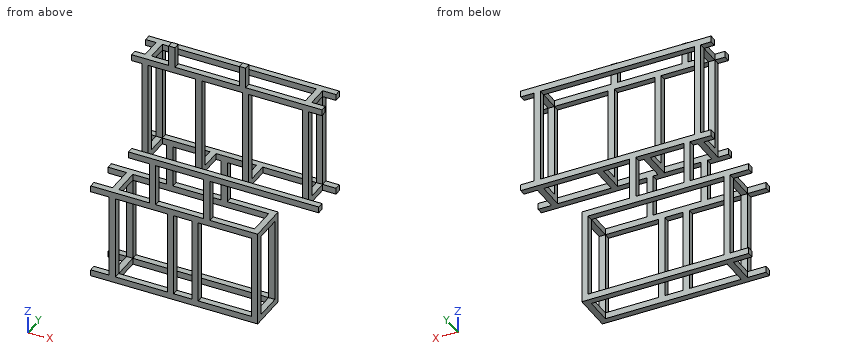
from build123d import *

# Parameters (mm, degrees)
SKETCH_1_W          = 30
SKETCH_1_H          = 450
SKETCH_1_W_2        = 910
SKETCH_1_H_2        = 30
EXTRUDE_1_DEPTH     = 30
SKETCH_2_W          = 30.109824799
SKETCH_2_H          = 30
SKETCH_2_W_2        = 30
EXTRUDE_2_DEPTH     = 100
SKETCH_3_W          = 49.418401049
SKETCH_3_H          = 30
SKETCH_3_W_2        = 30
SKETCH_3_W_3        = 910
SKETCH_3_H_2        = 450
EXTRUDE_3_DEPTH     = 30
SKETCH_4_W          = 850
SKETCH_4_H          = 30
SKETCH_4_W_2        = 30
SKETCH_4_H_2        = 400
EXTRUDE_4_DEPTH     = 30
SKETCH_5_W          = 30
SKETCH_5_H          = 30
EXTRUDE_5_DEPTH     = 130
SKETCH_6_W          = 88.479210194
SKETCH_6_H          = 30
SKETCH_6_W_2        = 30
SKETCH_6_H_2        = 400
SKETCH_6_W_3        = 850
EXTRUDE_6_DEPTH     = 30
SKETCH_8_W          = 736.515263892
SKETCH_8_H          = 30
SKETCH_8_W_2        = 64.066335059
SKETCH_8_W_3        = 49.418401049
CUT_EXTRUDE_2_DEPTH = 30
SKETCH_9_W          = 910
SKETCH_9_H          = 30
EXTRUDE_7_DEPTH     = 30
SKETCH_12_W         = 30
SKETCH_12_H         = 130
EXTRUDE_8_DEPTH     = 30
SKETCH_13_W         = 30
SKETCH_13_H         = 200
EXTRUDE_9_DEPTH     = 30
SKETCH_14_W         = 30
SKETCH_14_H         = 200
EXTRUDE_10_DEPTH    = 30
SKETCH_15_W         = 489.531957018
SKETCH_15_H         = 254.722560686
CUT_EXTRUDE_3_DEPTH = 51.972649134
SKETCH_16_W         = 30
SKETCH_16_H         = 30
EXTRUDE_11_DEPTH    = 100


with BuildPart() as part:
    # Sketch 1 → Extrude 1 (new body)
    with BuildSketch(Plane(origin=(0, 0, 0), x_dir=(1, 0, 0), z_dir=(0, 1, 0))):
        with Locations((64.418401049, 255)):
            Rectangle(SKETCH_1_W, SKETCH_1_H)
        with Locations((455, 15)):
            Rectangle(SKETCH_1_W_2, SKETCH_1_H_2)
        with Locations((321.408548695, 255)):
            Rectangle(SKETCH_1_W, SKETCH_1_H)
        with Locations((544.693031268, 255)):
            Rectangle(SKETCH_1_W, SKETCH_1_H)
        with Locations((830.933664941, 255)):
            Rectangle(SKETCH_1_W, SKETCH_1_H)
        Polygon((0, 480), (49.418401049, 480), (79.418401049, 480), (306.408548695, 480), (336.408548695, 480), (529.693031268, 480), (559.693031268, 480), (815.933664941, 480), (845.933664941, 480), (910, 480), (910, 510), (0, 510), align=None)
    extrude(amount=EXTRUDE_1_DEPTH)

    # Sketch 2 → Extrude 2 (add)
    with BuildSketch(Plane(origin=(0, 30, 0), x_dir=(1, 0, 0), z_dir=(0, 1, 0))):
        with Locations((64.473313449, 15)):
            Rectangle(SKETCH_2_W, SKETCH_2_H)
        with Locations((830.933664941, 15)):
            Rectangle(SKETCH_2_W_2, SKETCH_2_H)
        with Locations((64.418401049, 495)):
            Rectangle(SKETCH_2_W_2, SKETCH_2_H)
        with Locations((830.933664941, 495)):
            Rectangle(SKETCH_2_W_2, SKETCH_2_H)
    extrude(amount=EXTRUDE_2_DEPTH)

    # Sketch 3 → Extrude 3 (add)
    with BuildSketch(Plane(origin=(0, 130, 0), x_dir=(1, 0, 0), z_dir=(0, 1, 0))):
        Polygon((910, 510), (79.418401049, 510), (79.418401049, 480), (79.528225848, 480), (815.933664941, 480), (845.933664941, 480), (910, 480), align=None)
        with Locations((24.709200525, 495)):
            Rectangle(SKETCH_3_W, SKETCH_3_H)
        with Locations((64.418401049, 495)):
            Rectangle(SKETCH_3_W_2, SKETCH_3_H)
        with Locations((455, 15)):
            Rectangle(SKETCH_3_W_3, SKETCH_3_H)
        Polygon((79.418401049, 480), (49.418401049, 480), (49.418401049, 30), (79.528225848, 30), (79.528225848, 480), align=None)
        with Locations((830.933664941, 255)):
            Rectangle(SKETCH_3_W_2, SKETCH_3_H_2)
    extrude(amount=EXTRUDE_3_DEPTH)

    # Sketch 8 → Cut-Extrude 2 (cut)
    with BuildSketch(Plane(origin=(0, 0, -510), x_dir=(-1, 0, 0), z_dir=(0, 0, -1))):
        with Locations((-447.676032995, 15)):
            Rectangle(SKETCH_8_W, SKETCH_8_H)
        with Locations((-877.966832471, 15)):
            Rectangle(SKETCH_8_W_2, SKETCH_8_H)
        with Locations((-24.709200525, 15)):
            Rectangle(SKETCH_8_W_3, SKETCH_8_H)
    extrude(amount=-CUT_EXTRUDE_2_DEPTH, mode=Mode.SUBTRACT)



with BuildPart() as body_2:
    # Sketch 4 → Extrude 4 (new body)
    with BuildSketch(Plane(origin=(0, 160, 0), x_dir=(1, 0, 0), z_dir=(0, 1, 0))):
        with Locations((245, 725)):
            Rectangle(SKETCH_4_W, SKETCH_4_H)
        with Locations((245, 1155)):
            Rectangle(SKETCH_4_W, SKETCH_4_H)
        with Locations((-76.520789806, 940)):
            Rectangle(SKETCH_4_W_2, SKETCH_4_H_2)
        with Locations((603.027350866, 940)):
            Rectangle(SKETCH_4_W_2, SKETCH_4_H_2)
    extrude(amount=-EXTRUDE_4_DEPTH)

    # Sketch 5 → Extrude 5 (add)
    with BuildSketch(Plane(origin=(0, 130, 0), x_dir=(-1, 0, 0), z_dir=(0, -1, 0))):
        with Locations((76.520789806, 725)):
            Rectangle(SKETCH_5_W, SKETCH_5_H)
        with Locations((-603.027350866, 725)):
            Rectangle(SKETCH_5_W, SKETCH_5_H)
        with Locations((-603.027350866, 1155)):
            Rectangle(SKETCH_5_W, SKETCH_5_H)
        with Locations((76.520789806, 1155)):
            Rectangle(SKETCH_5_W, SKETCH_5_H)
    extrude(amount=EXTRUDE_5_DEPTH)

    # Sketch 6 → Extrude 6 (add)
    with BuildSketch(Plane(origin=(0, 0, 0), x_dir=(-1, 0, 0), z_dir=(0, -1, 0))):
        Polygon((-670, 710), (61.520789806, 710), (61.520789806, 740), (-186.822629959, 740), (-216.822629959, 740), (-303.86127731, 740), (-333.86127731, 740), (-588.027350866, 740), (-618.027350866, 740), (-670, 740), align=None)
        with Locations((135.760394903, 725)):
            Rectangle(SKETCH_6_W, SKETCH_6_H)
        with Locations((76.520789806, 725)):
            Rectangle(SKETCH_6_W_2, SKETCH_6_H)
        with Locations((76.520789806, 940)):
            Rectangle(SKETCH_6_W_2, SKETCH_6_H_2)
        with Locations((-201.822629959, 940)):
            Rectangle(SKETCH_6_W_2, SKETCH_6_H_2)
        with Locations((-318.86127731, 940)):
            Rectangle(SKETCH_6_W_2, SKETCH_6_H_2)
        with Locations((-603.027350866, 940)):
            Rectangle(SKETCH_6_W_2, SKETCH_6_H_2)
        with Locations((-245, 1155)):
            Rectangle(SKETCH_6_W_3, SKETCH_6_H)
    extrude(amount=EXTRUDE_6_DEPTH)


with BuildPart() as body_3:
    # Sketch 9 → Extrude 7 (new body)
    with BuildSketch(Plane(origin=(0, -30, 0), x_dir=(-1, 0, 0), z_dir=(0, -1, 0))):
        with Locations((-455, 495)):
            Rectangle(SKETCH_9_W, SKETCH_9_H)
    extrude(amount=-EXTRUDE_7_DEPTH)


with BuildPart() as part_1:
    add(part.part)

    add(body_3.part)  # Extrude 8 merges body 3
    # Sketch 12 → Extrude 8 (add)
    with BuildSketch(Plane(origin=(0, 0, -510), x_dir=(-1, 0, 0), z_dir=(0, 0, -1))):
        with Locations((-544.693031268, 65)):
            Rectangle(SKETCH_12_W, SKETCH_12_H)
        with Locations((-321.408548695, 65)):
            Rectangle(SKETCH_12_W, SKETCH_12_H)
    extrude(amount=-EXTRUDE_8_DEPTH)


    add(body_2.part)  # Extrude 9 merges body 2
    # Sketch 13 → Extrude 9 (add)
    with BuildSketch(Plane(origin=(0, -30, 0), x_dir=(-1, 0, 0), z_dir=(0, -1, 0))):
        with Locations((-115, 610)):
            Rectangle(SKETCH_13_W, SKETCH_13_H)
        with Locations((-375, 610)):
            Rectangle(SKETCH_13_W, SKETCH_13_H)
    extrude(amount=-EXTRUDE_9_DEPTH)

    # Sketch 14 → Extrude 10 (add)
    with BuildSketch(Plane(origin=(0, 160, 0), x_dir=(1, 0, 0), z_dir=(0, 1, 0))):
        with Locations((115, 610)):
            Rectangle(SKETCH_14_W, SKETCH_14_H)
        with Locations((375, 610)):
            Rectangle(SKETCH_14_W, SKETCH_14_H)
    extrude(amount=-EXTRUDE_10_DEPTH)

    # Sketch 15 → Cut-Extrude 3 (cut)
    with BuildSketch(Plane(origin=(670, 0, 0), x_dir=(0, 0, -1), z_dir=(1, 0, 0))):
        with Locations((948.415249447, 56.198014116)):
            Rectangle(SKETCH_15_W, SKETCH_15_H)
    extrude(amount=-CUT_EXTRUDE_3_DEPTH, mode=Mode.SUBTRACT)

    # Sketch 16 → Extrude 11 (add)
    with BuildSketch(Plane.XY):
        with Locations((192.165247783, 15)):
            Rectangle(SKETCH_16_W, SKETCH_16_H)
        with Locations((529.958608766, 15)):
            Rectangle(SKETCH_16_W, SKETCH_16_H)
    extrude(amount=EXTRUDE_11_DEPTH)


solid = part_1.part
Work out the finished part from the listing and answer in its coordinate system (mm). Round coordinates to 2 decimals unless told otherwise and drop trailing zeros. Write each loop counter-clockwise with the first axis right and the second up, starting at its lowest first coordinate (ties: lowest second). Pieces come first, ordered by that corner, then holes. Notation, with made-up numbers: (89.25, 73) - (96.25, 73) arc R21 ccw to (96.25, 97) - close; hole circle Ø6 at (56.25, 57.5). An arc over 180 degrees is marked (long way). Answer in a Markdown table with one row per item. Add a question column.
1. A cutting plane is placed at C-C, the plane z = -607. Determine the outline of the cut face in (x, y).
2. Given pin 1 (15 mm diameter, centred on x = 283, y = 138.5, fed in from +Z); pin 2 (15 mm diameter, centred on y = 145, z = -867, fed in from -X); pin 3 (5 mm diameter, centred on x = 266, y = 20.5, fed in from -Z), each flat-ended and moving along its own axis, determine where each tip first touches the part or whether it passes through.
3. Find the intervals of material crossed by line 1 along X through (y, z) = (-0.5, -902); line 2 along Z through (x, y) = (25, -20); line 3 along X through (y, z) = (22, -439.5), in increasing order. Write a range as from..to.
4. A cutting plane is placed at B-B, the plane x = 709. Determine the outline of the cut face in (y, z).
5. A cutting plane is placed at A-A, the plane z = -757. Determine the outline of the cut face in (x, y), and give its area (3 significant figures).
6. A cutting plane is placed at D-D, the plane y = 112. Count the separate pieces of the cut face and the enclosed holes in it, and give its area (3 significant figures).
Worked out:
| question | item | result |
|---|---|---|
| 1 | outline | (100, -30) - (130, -30) - (130, 0) - (100, 0) - close; (100, 130) - (130, 130) - (130, 160) - (100, 160) - close; (360, -30) - (390, -30) - (390, 0) - (360, 0) - close; (360, 130) - (390, 130) - (390, 160) - (360, 160) - close |
| 2 | pin 1 | z = 0 |
| 2 | pin 2 | x = -91.52 |
| 2 | pin 3 | z = -30 |
| 3 | line 1 | -91.52..-61.52, 186.82..216.82, 303.86..333.86, 588.03..618.03 |
| 3 | line 2 | -1170..-1140, -740..-710, -510..-480 |
| 3 | line 3 | 49.42..79.42, 306.41..336.41, 529.69..559.69, 815.93..845.93 |
| 4 | outline | (-30, -510) - (0, -510) - (0, -480) - (-30, -480) - close; (0, -30) - (30, -30) - (30, 0) - (0, 0) - close; (130, -510) - (160, -510) - (160, -480) - (130, -480) - close; (130, -30) - (160, -30) - (160, 0) - (130, 0) - close |
| 5 | outline | (-91.52, -30) - (-61.52, -30) - (-61.52, 0) - (-91.52, 0) - close; (-91.52, 130) - (-61.52, 130) - (-61.52, 160) - (-91.52, 160) - close; (186.82, -30) - (216.82, -30) - (216.82, 0) - (186.82, 0) - close; (303.86, -30) - (333.86, -30) - (333.86, 0) - (303.86, 0) - close; (588.03, -30) - (618.03, -30) - (618.03, 0) - (588.03, 0) - close; (588.03, 130) - (618.03, 130) - (618.03, 160) - (588.03, 160) - close |
| 5 | area | 5,400 mm^2 |
| 6 | separate pieces | 10 |
| 6 | enclosed holes | 0 |
| 6 | area | 9,000 mm^2 |
